Geometry check sheet. Reference: the model listing, model coordinates, mm. A direction names the side the tool comes from. Round coordinates to 2 decimals unless told otherwise and drop trailing zeros. Order: outer loops, then holes, each group sorted by start corner. A loop starts at its lowest first (then second) coordinate and runs counter-clockwise, first axis right, second up. Notation, with made-up numbers: (-31.5, 67) - (-14.5, 67) arc R20 ccw to (-14.5, 98) - close; hole circle Ø5 at (68.25, -23.5). An arc over 180 degrees is marked (long way). One line per question, with ' | ' between items. Start each with the question number.
Q1. Material ranges on line 1 along Y through (x, z) = (5.75, 5.5); line 2 along Y through (x, z) = (9.5, -5); line 3 along X through (y, z) = (-0.25, 18), recorded low to high.
Q2. Sectioned sample at D-D, the plane y = 6.75. Enter the section's corners in (x, z).
Q3. Mould release check, pull along Y, two halves, no side actions. Record for faces 3 (the face through (11.554, -0.254, 0.652)), 4 (the face through (10.5, 0.1, -19.05)), 5 (the face through (10.285, -0.226, 0.652)): +Y half, -Y half, draft (parallel to the pull), parting line (faces both ways), or undercut.
Q4. Sectioned sample at A-A, the plane x = 8.5. Enter the section's corners in (y, z), then the cut area to 3 significant figures.
Q5. Sectioned sample at C-C, the plane z = 6. Enter the section's corners in (x, y), then the cut area to 3 significant figures.
Q6. Tool access check on faces 1 (the face through (3.95, 0.14, 19.26)), 2 (the face through (0, 11, 1)). Record the directions out of +Z, -Z, +X, -X, +Y, -Y that give a thin tool (end or side, any length) a straight path to the whole face; none if there is none.
Q7. Sectioned sample at B-B, the plane y = 0. Enter the section's corners in (x, z), then the cut area to 3 significant figures.
Q8. Gauge pin test, flat ends, axial feed: P1, Ø1.5, axis at y = -4, z = 6.5, coming from the +X side; P2, Ø4, axis at y = 5, z = -11.5, coming from the -X side; P3, Ø6, axis at x = 2, z = 9.5, coming from the +Y side; P4, Ø5, axis at y = -3.5, z = -3, coming from the +X side. Record the tip position at first contact, or that the pin passes through.
```python
from build123d import *

# Parameters (mm, degrees)
F1_DEPTH    = 19.05
F3_DEPTH    = 0.75946
F4_T4_DEPTH = 76.9415838332
F4_S5_R     = 10.287
F4_T6_DEPTH = 40


# Not quite as in the source:
# - a fillet or chamfer that OpenCascade refuses, or shapes differently, is made with other operations: its cross-section is extruded or revolved along the edge and cut away or added


with BuildPart() as f1:
    # F0 (on Top) → F1 (new body, symmetric)
    with BuildSketch(Plane.XY):
        with BuildLine():
            ThreePointArc((0, 10.287), (10.287, 0), (0, -10.287))
            Line((0, -10.287), (0, -11.557))
            ThreePointArc((0, -11.557), (11.557, 0), (0, 11.557))
            Line((0, 11.557), (0, 10.287))
        make_face()
    extrude(amount=F1_DEPTH, both=True)

    # F2 (on face) → F3 (join, symmetric)
    with BuildSketch(Plane.XY.offset(19.05)):
        with BuildLine():
            Line((0, 11.557), (0, -11.557))
            ThreePointArc((0, -11.557), (11.557, 0), (0, 11.557))
        make_face()
    extrude(amount=F3_DEPTH, both=True)

    # F4: chamfer of 1.524 x 10.8438234569 on 1 edges, made by hand


with BuildPart() as f4_tool2:
    # F4_s3 → F4_t4 (new body)
    with BuildSketch(Plane.XZ.offset(-38.4707919166)):
        Polygon((0, 19.81454), (10.8438234569, 18.29054), (0, 18.29054), align=None)
    extrude(amount=F4_T4_DEPTH)

    # F4_s5 → F4_t6 (intersect, symmetric)
    with BuildSketch(Plane.XY.offset(19.1)):
        Circle(F4_S5_R)
    extrude(amount=F4_T6_DEPTH, both=True, mode=Mode.INTERSECT)


with BuildPart() as f1_1:
    add(f1.part)

    # F4_t1: cut F4_tool2
    add(f4_tool2.part, mode=Mode.SUBTRACT)


solid = f1_1.part
```
Determined:
1) line 1: y = -10.03 to -8.53, 8.53 to 10.03 | line 2: y = -6.58 to -3.95, 3.95 to 6.58 | line 3: x = 10.28 to 11.55
2) outline: (0.04, 19.81) - (7.76, 18.72) - (7.76, -19.05) - (9.38, -19.05) - (9.38, 19.81) - close
3) face 3: parting line | face 4: draft | face 5: undercut
4) outline: (-7.83, -19.05) - (-5.79, -19.05) - (-5.79, 18.62) - (5.79, 18.62) - (5.79, -19.05) - (7.83, -19.05) - (7.83, 19.81) - (-7.83, 19.81) - close | area: 172 mm2
5) outline: (0, -11.56) arc R11.56 ccw to (0, 11.56) - (0, 10.29) arc R10.29 cw to (0, -10.29) - close | area: 43.6 mm2
6) face 1: -Z, -X | face 2: +Z, -Z, -X, +Y, -Y
7) outline: (0.04, 19.81) - (10.29, 18.37) - (10.29, -19.05) - (11.56, -19.05) - (11.56, 19.81) - close | area: 56.7 mm2
8) P1: stops at x = 11.09 | P2: stops at x = 7.54 | P3: stops at y = 11.56 | P4: stops at x = 11.51
